Here's how the part is built. I have some questions about the finished solid (model axes, mm). A direction names the side the tool comes from. Round coordinates to 2 decimals unless told otherwise and drop trailing zeros. Write each loop counter-clockwise with the first axis right and the second up, starting at its lowest first coordinate (ties: lowest second). Pieces come first, ordered by that corner, then holes. Notation, with made-up numbers: (89.25, 49) -> (107.25, 49) arc R24 cw to (107.25, 83) -> close; hole circle Ø6 at (53, 30.5). An arc over 180 degrees is marked (long way). Put each result on its own line as item: value. Start each with the question number.
1. Suppose I cut it at C-C (y = -14). Please give me the cut outline in (x, z), then the cut area to 3 significant figures.
2. Suppose I cut it at D-D (x = 1.1). Please give me the cut outline in (y, z).
3. Suppose I cut it at B-B (z = 1.2). Please give me the cut outline in (x, y), then the cut area to 3 significant figures.
4. For pin 1 (1.3 mm diameter, centred on x = -0.5, y = -3, fed in from +Z); pin 2 (0.6 mm diameter, centred on x = 0.5, z = 2, fed in from +Y), each with a flat end and sliding along its axis, tell me the tip position at first contact or that it passes through.
5. Which directions (+Z, -Z, +X, -X, +Y, -Y) give clear straight access to the entire face, cutting with the end or side of a thin tool? Please do faces 1 (the face through (0, 0, 0)), 2 (the face through (0, -2, 1.5)), 3 (the face through (0, -13, 1.5)).
6. I need wall thicknesses on probe 1 along X at (y, z) = (-14.5, -1.5); probe 2 along X at (y, z) = (-2, -0.7); probe 3 along Z at (x, y) = (-0.5, -9). Which ranges of each line are inside material? Lowest first, please. Write a range as from..to.
7. Suppose I cut it at A-A (x = 0). Please give me the cut outline in (y, z).
```python
from build123d import *
from build123d import SkipClean  # not in build123d's __all__

# Parameters (mm, degrees)
F1_DEPTH = 16
F3_START = -5
F2_R     = 2
F3_DEPTH = 6


with BuildPart() as f1:
    # F0 (on Front) → F1 (new body)
    with BuildSketch(Plane.XZ):
        with BuildLine():
            ThreePointArc((-1.3228756555, 1.5), (-0.8228756555, -1.8228756555), (2, 0))
            ThreePointArc((2, 0), (1.8228756555, 0.8228756555), (1.3228756555, 1.5))
            Line((1.3228756555, 1.5), (-1.3228756555, 1.5))
        make_face()
    extrude(amount=F1_DEPTH)

    # F2 (on face) → F3 (join)
    with BuildSketch(Plane.XZ.offset(16).offset(F3_START)):
        Circle(F2_R)
    with SkipClean():  # cleaning this boolean's faces spoils the solid; the shape is the same uncleaned
        extrude(amount=-F3_DEPTH)


solid = f1.part
```
Verdict:
1. outline: (-1.32, 1.5) arc R2 ccw (long way) to (1.32, 1.5) -> close
1. area: 11.7 mm^2
2. outline: (-16, -1.67) -> (0, -1.67) -> (0, 1.5) -> (-5, 1.5) -> (-5, 1.67) -> (-11, 1.67) -> (-11, 1.5) -> (-16, 1.5) -> close
3. outline: (-1.6, -16) -> (1.6, -16) -> (1.6, 0) -> (-1.6, 0) -> close
3. area: 51.2 mm^2
4. pin 1: stops at z = 1.5
4. pin 2: stops at y = -5
5. face 1: +Z, -Z, +X, -X, +Y
5. face 2: +Z, +X, -X, +Y
5. face 3: +Z, +X, -X, -Y
6. probe 1: x = -1.32..1.32
6. probe 2: x = -1.87..1.87
6. probe 3: z = -1.94..1.94
7. outline: (-16, -2) -> (0, -2) -> (0, 1.5) -> (-5, 1.5) -> (-5, 2) -> (-11, 2) -> (-11, 1.5) -> (-16, 1.5) -> close
